from build123d import *

# Parameters (mm, degrees)
SKETCH1_R           = 1.5
SKETCH1_W           = 11
SKETCH1_H           = 2
BOSS_EXTRUDE1_DEPTH = 2
SKETCH1_3_W         = 11
SKETCH1_3_H         = 2
BOSS_EXTRUDE2_DEPTH = 20
FILLET2_R           = 2
FILLET3_R           = 1


with BuildPart() as part:
    # Sketch1 → Boss-Extrude1 (new body)
    # profile 1 of 7: a face of its own
    with BuildSketch(Plane(origin=(0, 0, 0), x_dir=(1, 0, 0), z_dir=(0, 1, 0))):
        Polygon((0, -6.315863562), (0, -2), (-3, -2), (-3, 13), (0, 13), (0, 17.315863562), (-7.816047118, 17.315863562), (-7.816047118, -6.315863562), align=None)
        with Locations(Location((-5, -3.5, 0), (0, 0, 270))):
            Circle(SKETCH1_R, mode=Mode.SUBTRACT)
        with Locations(Location((-5, 14.5, 0), (0, 0, 270))):
            Circle(SKETCH1_R, mode=Mode.SUBTRACT)
    # profile 2 of 7: a face of its own
    with BuildSketch(Plane(origin=(0, 0, 0), x_dir=(1, 0, 0), z_dir=(0, 1, 0))):
        Polygon((0, -2), (0, 0), (0, 11), (0, 13), (-3, 13), (-3, -2), align=None)
    # profile 3 of 7: a face of its own
    with BuildSketch(Plane(origin=(0, 0, 0), x_dir=(1, 0, 0), z_dir=(0, 1, 0))):
        Polygon((0, -6.315863562), (0, -2), (-3, -2), (-3, 13), (0, 13), (0, 17.315863562), (-7.816047118, 17.315863562), (-7.816047118, -6.315863562), align=None)
        with Locations(Location((-5, -3.5, 0), (0, 0, 270))):
            Circle(SKETCH1_R, mode=Mode.SUBTRACT)
        with Locations(Location((-5, 14.5, 0), (0, 0, 270))):
            Circle(SKETCH1_R, mode=Mode.SUBTRACT)
    # profile 4 of 7: a face of its own
    with BuildSketch(Plane(origin=(0, 0, 0), x_dir=(1, 0, 0), z_dir=(0, 1, 0))):
        Polygon((0, -6.315863562), (0, -2), (-3, -2), (-3, 13), (0, 13), (0, 17.315863562), (-7.816047118, 17.315863562), (-7.816047118, -6.315863562), align=None)
        with Locations(Location((-5, -3.5, 0), (0, 0, 270))):
            Circle(SKETCH1_R, mode=Mode.SUBTRACT)
        with Locations(Location((-5, 14.5, 0), (0, 0, 270))):
            Circle(SKETCH1_R, mode=Mode.SUBTRACT)
    # profile 5 of 7: a face of its own
    with BuildSketch(Plane(origin=(0, 0, 0), x_dir=(1, 0, 0), z_dir=(0, 1, 0))):
        with Locations((5.5, -1)):
            Rectangle(SKETCH1_W, SKETCH1_H)
    # profile 6 of 7: a face of its own
    with BuildSketch(Plane(origin=(0, 0, 0), x_dir=(1, 0, 0), z_dir=(0, 1, 0))):
        Polygon((0, -2), (0, 0), (0, 11), (0, 13), (-3, 13), (-3, -2), align=None)
    # profile 7 of 7: a face of its own
    with BuildSketch(Plane(origin=(0, 0, 0), x_dir=(1, 0, 0), z_dir=(0, 1, 0))):
        with Locations((5.5, 12)):
            Rectangle(SKETCH1_W, SKETCH1_H)
    extrude(amount=BOSS_EXTRUDE1_DEPTH)

    # Sketch1_3 → Boss-Extrude2 (add)
    with BuildSketch(Plane(origin=(0, 0, 0), x_dir=(1, 0, 0), z_dir=(0, 1, 0))):
        Polygon((0, -2), (0, 0), (0, 11), (0, 13), (-3, 13), (-3, -2), align=None)
        with Locations((5.5, -1)):
            Rectangle(SKETCH1_3_W, SKETCH1_3_H)
        with Locations((5.5, 12)):
            Rectangle(SKETCH1_3_W, SKETCH1_3_H)
    extrude(amount=BOSS_EXTRUDE2_DEPTH)

    # Fillet2
    fillet2_edges = [part.edges().sort_by_distance(p)[0] for p in [
        (0, 1, 6.315863562),
        (-7.816047118, 1, 6.315863562),
        (-7.816047118, 1, -17.315863562),
        (0, 1, -17.315863562),
        (0, 1, -13),
        (0, 1, 2),
        (-3, 11, -13),
        (-3, 11, 2),
    ]]
    fillet(fillet2_edges, radius=FILLET2_R)

    # Fillet3
    fillet3_edges = [part.edges().sort_by_distance(p)[0] for p in [
        (0.5, 2, 2),
        (-2.414213562, 2, 1.414213562),
        (-2.414213562, 2, -12.414213562),
        (-3, 2, -5.5),
        (0.5, 2, -13),
    ]]
    fillet(fillet3_edges, radius=FILLET3_R)


solid = part.part
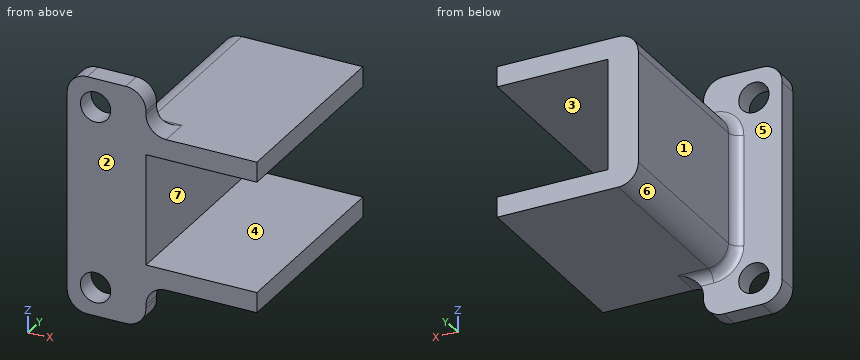
Verification items for the finished model (mm, model axes). Face numbers are marked on the shaded views. A direction names the side the tool comes from. Coordinates: 2 decimals unless noted, no trailing zeros. Order: outer loops, then holes, each group sorted by start corner. A loop starts at its lowest first (then second) coordinate and runs counter-clockwise, first axis right, second up.
1. Sectioned sample at C-C, the plane x = 1.5. Record the cut outline in (y, z), and give its area (3 significant figures).
Results found:
outline: (0, -13.06) - (2.65, -13.06) arc R1 cw to (3, -13) - (20, -13) - (20, -11) - (0, -11) - close; (0, 0) - (20, 0) - (20, 2) - (3, 2) arc R1 cw to (2.65, 2.06) - (0, 2.06) - close
area: 80.4 mm2
2. Sectioned sample at A-A, the plane x = -5. Record the cut outline in (y, z), and give its area (3 significant figures).
Results found:
outline: (0, -17.32) - (2, -17.32) - (2, -16) - (0, -16) - close; (0, -13) - (2, -13) - (2, 2) - (0, 2) - close; (0, 5) - (2, 5) - (2, 6.32) - (0, 6.32) - close
area: 35.3 mm2
3. Release check for a two-part mould opening along Z. For the marked faces 4, 5, 6 and 7 record: +Z half, -Z half, draft (parallel to the pull), parting line (faces both ways), or undercut.
Results found:
face 4: undercut
face 5: draft
face 6: -Z half
face 7: undercut
4. Set-up check for the marked faces 1, 2 and 3: record each of +Z, -Z, +X, -X, +Y, -Y from which the full face is reachable in a straight line by a thin tool's end or side.
Results found:
face 1: +Z, -Z, -X, +Y
face 2: +Z, -Z, +X, -X, -Y
face 3: +X, +Y, -Y
5. Sectioned sample at D-D, the plane y = 13. Record the cut outline in (x, z), and give its area (3 significant figures).
Results found:
outline: (-3, -11) arc R2 ccw to (-1, -13) - (11, -13) - (11, -11) - (0, -11) - (0, 0) - (11, 0) - (11, 2) - (-1, 2) arc R2 ccw to (-3, 0) - close
area: 87.3 mm2
6. Sectioned sample at B-B, the plane z = -1.5. Record the cut outline in (x, y).
Results found:
outline: (-7.82, 0) - (0, 0) - (0, 20) - (-3, 20) - (-3, 3) arc R1 cw to (-4, 2) - (-7.82, 2) - close
7. Scan lines: line 1 (Z direction, x = 5, y = 1.5); line 2 (X direction, y = 10.25, z = -7.5); line 3 (Y direction, x = -4.5, z = 2). Record each from-to range of solid material in increasing order.
Results found:
line 1: z = -13 to -11, 0 to 2
line 2: x = -3 to 0
line 3: y = 0 to 2
8. Go/stop test with flat-tipped pins: pin 1 Ø3.5 at (y, z) = (14, -8) entering from -X; pin 2 Ø1.5 at (y, z) = (12, -5) entering from +X; pin 3 Ø3.5 at (x, y) = (4.5, 8) entering from +Z. Record where each tip stops, or that it passes through.
Results found:
pin 1: stops at x = -3
pin 2: stops at x = 0
pin 3: stops at z = 2
